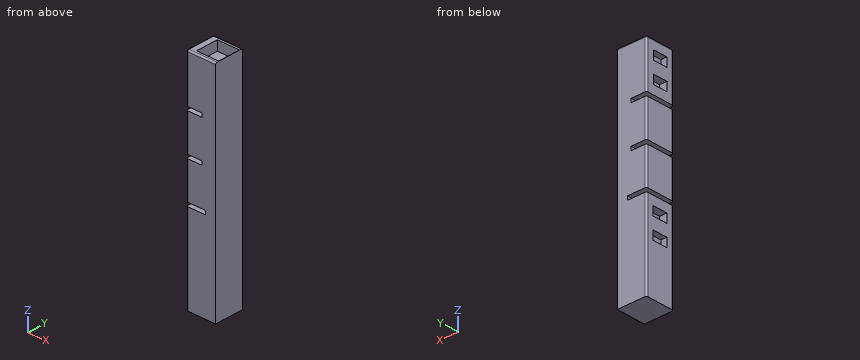
Autodesk Fusion 360 part; units mm, degrees
sketch "Sketch1" plane through (0, 0, 0) normal (0, 0, 1) x (1, 0, 0)
  line L0 (9.925, 9.925) -> (-9.925, 9.925)
  line L1 (-9.925, 9.925) -> (-9.925, -9.925)
  line L2 (-9.925, -9.925) -> (9.925, -9.925)
  line L3 (9.925, -9.925) -> (9.925, 9.925)
  line L4 (9.925, 9.925) -> (-9.925, -9.925) construction
  line L5 (-9.925, 9.925) -> (9.925, -9.925) construction
  dimension "d1" = 19.85
  dimension "d2" = 19.85
extrude "Extrude1" add sketch "Sketch1" along normal blind 150
sketch "Sketch2" plane through (0, -9.925, 0) normal (0, -1, 0) x (1, 0, 0)
  line L0 (-9.925, 0) -> (9.925, 0)
  line L1 (9.925, 0) -> (9.925, 150)
  line L2 (9.925, 150) -> (-9.925, 150)
  line L3 (-9.925, 150) -> (-9.925, 0)
  line L4 (-9.925, 62.54) -> (2.925, 62.54)
  line L5 (2.925, 62.54) -> (2.925, 60)
  line L6 (2.925, 60) -> (-9.925, 60)
  line L7 (-9.925, 60) -> (-9.925, 62.54)
  line L8 (-9.925, 90.08) -> (0.535, 90.08)
  line L9 (0.535, 90.08) -> (0.535, 87.54)
  line L10 (0.535, 87.54) -> (-9.925, 87.54)
  line L11 (-9.925, 87.54) -> (-9.925, 90.08)
  line L12 (-9.925, 117.62) -> (0.535, 117.62)
  line L13 (0.535, 117.62) -> (0.535, 115.08)
  line L14 (0.535, 115.08) -> (-9.925, 115.08)
  line L15 (-9.925, 115.08) -> (-9.925, 117.62)
  dimension "d5" = 12.85
  dimension "d6" = 2.54
  dimension "d7" = 60
  dimension "d8" = 10.46
  dimension "d9" = 2.54
  dimension "d10" = 25
  dimension "d11" = 10.46
  dimension "d12" = 2.54
  dimension "d13" = 25
extrude "Extrude2" cut sketch "Sketch2" against normal blind 30 contours L3 L4 L5 L6 L7 | L3 L8 L9 L10 L11 | L3 L12 L13 L14 L15
fillet "Fillet1" radius 1 8 edges at (-9.925, -9.925, 133.81) (-9.925, -9.925, 102.58) (-9.925, -9.925, 75.04) (-9.925, -9.925, 30) (-9.925, 9.925, 133.81) (-9.925, 9.925, 102.58) (-9.925, 9.925, 75.04) (-9.925, 9.925, 30)
fillet "Fillet2" radius 1 5 edges at (0.5, 9.925, 150) (-9.6321, 9.6321, 150) (-9.925, 0, 150) (-9.6321, -9.6321, 150) (0.5, -9.925, 150)
sketch "Sketch3" plane through (-9.925, 0, 0) normal (-1, 0, 0) x (0, -1, 0)
  line L0 (8.925, 149) -> (-8.925, 149)
  line L1 (-8.925, 149) -> (-8.925, 117.62)
  line L2 (-8.925, 117.62) -> (8.925, 117.62)
  line L3 (8.925, 117.62) -> (8.925, 149)
  line L4 (5.075, 129.62) -> (-4.925, 129.62)
  line L5 (-4.925, 129.62) -> (-4.925, 123.62)
  line L6 (-4.925, 123.62) -> (5.075, 123.62)
  line L7 (5.075, 123.62) -> (5.075, 129.62)
  line L8 (5.075, 129.62) -> (-4.925, 123.62) construction
  line L9 (-4.925, 129.62) -> (5.075, 123.62) construction
  line L10 (-4.9698, 54) -> (5.0302, 54)
  line L11 (5.0302, 54) -> (5.0302, 48)
  line L12 (5.0302, 48) -> (-4.9698, 48)
  line L13 (-4.9698, 48) -> (-4.9698, 54)
  line L14 (-4.9698, 54) -> (5.0302, 48) construction
  line L15 (5.0302, 54) -> (-4.9698, 48) construction
  line L16 (8.925, 60) -> (-8.925, 60)
  point P0 (0.075, 126.62)
  point P1 (0.0302, 51)
  dimension "d20" = 10
  dimension "d21" = 6
  dimension "d22" = 3.85
  dimension "d23" = 6
  dimension "d24" = 6
  dimension "d25" = 10
  dimension "d26" = 6
extrude "Extrude3" cut sketch "Sketch3" against normal blind 5 contours L4 L5 L6 L7 | L10 L11 L12 L13
sketch "Sketch4" plane through (0, 0, 150) normal (0, 0, 1) x (-1, 0, 0)
  line L0 (8.925, 8.925) -> (-9.925, 8.925)
  line L1 (-9.925, 8.925) -> (-9.925, -8.925)
  line L2 (-9.925, -8.925) -> (8.925, -8.925)
  line L3 (8.925, -8.925) -> (8.925, 8.925)
  line L4 (-9.775, -7.625) -> (5.225, -7.625)
  line L5 (5.225, -7.625) -> (5.225, 7.575)
  line L6 (5.225, 7.575) -> (-9.775, 7.575)
  line L7 (-9.775, 7.575) -> (-9.775, -7.625)
  line L8 (-9.775, -7.625) -> (5.225, 7.575) construction
  line L9 (5.225, -7.625) -> (-9.775, 7.575) construction
  point P0 (-2.275, -0.025)
  dimension "d29" = 15
  dimension "d30" = 15.2
  dimension "d31" = 1.3
  dimension "d32" = 3.7
extrude "Extrude4" cut sketch "Sketch4" against normal blind 6.6 contours L4 L5 L6 L7
sketch "Sketch7" plane through (-9.925, 0, 0) normal (-1, 0, 0) x (0, -1, 0)
  line L0 (-4.925, 129.62) -> (5.075, 129.62)
  line L1 (5.075, 129.62) -> (5.075, 123.62)
  line L2 (5.075, 123.62) -> (-4.925, 123.62)
  line L3 (-4.925, 123.62) -> (-4.925, 129.62)
  line L4 (8.925, 149) -> (-8.925, 149)
  line L5 (-8.925, 149) -> (-8.925, 117.62)
  line L6 (-8.925, 117.62) -> (8.925, 117.62)
  line L7 (8.925, 117.62) -> (8.925, 149)
  line L8 (5.075, 143.62) -> (-4.925, 143.62)
  line L9 (-4.925, 143.62) -> (-4.925, 137.62)
  line L10 (-4.925, 137.62) -> (5.075, 137.62)
  line L11 (5.075, 137.62) -> (5.075, 143.62)
  line L12 (5.075, 143.62) -> (-4.925, 137.62) construction
  line L13 (-4.925, 143.62) -> (5.075, 137.62) construction
  line L14 (5.0197, 34) -> (-4.9803, 34)
  line L15 (-4.9803, 34) -> (-4.9803, 40)
  line L16 (-4.9803, 40) -> (5.0197, 40)
  line L17 (5.0197, 40) -> (5.0197, 34)
  line L18 (5.0197, 34) -> (-4.9803, 40) construction
  line L19 (-4.9803, 34) -> (5.0197, 40) construction
  line L20 (5.0302, 48) -> (-4.9698, 48)
  point P0 (0.075, 140.62)
  point P1 (0.0197, 37)
  dimension "d45" = 8
  dimension "d46" = 3.85
  dimension "d47" = 6
  dimension "d48" = 10
  dimension "d49" = 6
  dimension "d50" = 8
extrude "Extrude6" cut sketch "Sketch7" against normal blind 4 contours L8 L9 L10 L11 | L14 L15 L16 L17
The listing builds one solid part. Answer for the finished solid, in the listing's coordinates (mm). Coordinates: 2 decimals unless noted, no trailing zeros. Write each loop counter-clockwise with the first axis right and the second up, starting at its lowest first coordinate (ties: lowest second). Pieces come first, ordered by that corner, then holes. Notation, with made-up numbers: (-36.5, 61.25) - (8.5, 61.25) arc R22 cw to (8.5, 92.25) - close; hole circle Ø7 at (78.5, -35). An arc over 180 degrees is marked (long way). Return JSON: item names as keys, results as strings. Group by question number.
1. A cutting plane is placed at B-B, the plane z = 50.5. Determine the outline of the cut face in (x, y) (3 decimals), plus the area to 3 significant figures.
2. Straight lines are drawn through the part: L1, parallel to Z at x = -5, y = -4.5; L2, parallel to Z at x = -5, y = -6.25; L3, parallel to Z at x = 2, y = -3.25. For each, find the intervals that lie inside material, in ascending order.
3. Given pin 1 (0.8 mm diameter, centred on y = -5, z = 61.5, fed in from -X) (3 decimals); pin 2 (4 mm diameter, centred on x = -2, y = -1.5, fed in from +Z), each flat-ended and moving along its own axis, determine where each tip first touches the part or whether it passes through.
4. A cutting plane is placed at A-A, the plane x = -1. Determine the outline of the cut face in (y, z) (3 decimals).
5. A cutting plane is placed at C-C, the plane x = 4.5. Determine the outline of the cut face in (y, z) (3 decimals).
Ans:
{
 "1": {"outline": "(-9.925, -8.925) arc R1 ccw to (-8.925, -9.925) - (9.925, -9.925) - (9.925, 9.925) - (-8.925, 9.925) arc R1 ccw to (-9.925, 8.925) - (-9.925, 4.97) - (-4.925, 4.97) - (-4.925, -5.03) - (-9.925, -5.03) - close", "area": "344 mm²"},
 "2": {"L1": "0 to 48, 54 to 60, 62.54 to 87.54, 90.08 to 115.08, 117.62 to 123.62, 129.62 to 143.4", "L2": "0 to 60, 62.54 to 87.54, 90.08 to 115.08, 117.62 to 143.4", "L3": "0 to 60, 62.54 to 143.4"},
 "3": {"pin 1": "x = 2.925", "pin 2": "z = 143.4"},
 "4": {"outline": "(-9.925, 0) - (9.925, 0) - (9.925, 60) - (-9.925, 60) - close; (-9.925, 62.54) - (9.925, 62.54) - (9.925, 87.54) - (-9.925, 87.54) - close; (-9.925, 90.08) - (9.925, 90.08) - (9.925, 115.08) - (-9.925, 115.08) - close; (-9.925, 117.62) - (9.925, 117.62) - (9.925, 149) arc R1 ccw to (8.925, 150) - (7.625, 150) - (7.625, 143.4) - (-7.575, 143.4) - (-7.575, 150) - (-8.925, 150) arc R1 ccw to (-9.925, 149) - close"},
 "5": {"outline": "(-9.925, 0) - (9.925, 0) - (9.925, 149) arc R1 ccw to (8.925, 150) - (7.625, 150) - (7.625, 143.4) - (-7.575, 143.4) - (-7.575, 150) - (-8.925, 150) arc R1 ccw to (-9.925, 149) - close"}
}
